The listing builds one solid part. Answer for the finished solid, in the listing's coordinates (mm). A direction names the side the tool comes from. Round coordinates to 2 decimals unless told otherwise and drop trailing zeros. Order: outer loops, then holes, each group sorted by start corner. A loop starts at its lowest first (then second) coordinate and runs counter-clockwise, first axis right, second up. Notation, with made-up numbers: M 53,32.5 L 81,32.5 A18 ccw 81,56.5 Z; hole C 76.25,82.5 d1. An arc over 180 degrees is marked long. Put each result on its own line as item: value. Start each with the question number.
1. The part is cut by section D-D (x = 92). Give the vertices of the cut face in (y, z).
2. The part is cut by section A-A (x = 58.5). Give the vertices of the cut face in (y, z).
3. Consider line 1 (Y direction, x = 32, z = -0.75); line 2 (X direction, y = 49, z = 20.75); line 3 (Z direction, x = 167.5, y = 57). Determine where each line is inside the solid, lowest interval first.
4. Which of the six approach directions +Z, -Z, +X, -X, +Y, -Y give full straight-line access (tool end or side, diameter ignored) to faces 1 (the face through (165.1, 23, 11)), 2 (the face through (-4, 55.88, 21)), 3 (the face through (172.72, 23, 13)), 4 (the face through (-7.62, 23, 13)), 5 (the face through (81, 20, -1.07))?
5. Each of these flat-tipped pins is pushed along its axis until it touches: pin 1 Ø1.2 at (x, z) = (129.5, -0.5) entering from +Y; pin 2 Ø6 at (x, y) = (-13, 12) entering from +Z; pin 3 Ø5 at (x, y) = (115.5, 75.5) entering from -Z; pin 4 Ø1 at (x, y) = (-5, 11) entering from -Z. Where does it stop, or does it pass through?
6. The part is cut by section C-C (y = 34). Give the vertices of the cut face in (x, z), then the cut area to 3 significant figures.
7. The part is cut by section B-B (z = 6.5). Give the vertices of the cut face in (x, y).
from build123d import *

# Parameters (mm, degrees)
SKETCH1_W           = 165.1
SKETCH1_H           = 55.88
BOSS_EXTRUDE1_DEPTH = 2.54
SKETCH1_3_W         = 7.62
SKETCH1_3_H         = 55.88
BOSS_EXTRUDE2_DEPTH = 20
BOSS_EXTRUDE3_DEPTH = 64.2
BOSS_EXTRUDE4_REACH = 127.654
SKETCH3_W           = 2.139816337
SKETCH3_H           = 2.547064604
SKETCH3_H_2         = 2.262901763
SKETCH3_W_2         = 1.069908168
SKETCH3_H_3         = 3.883558818
BOSS_EXTRUDE5_DEPTH = 19.05
BOSS_EXTRUDE6_DEPTH = 2.54
SKETCH6_W           = 26.96027589
SKETCH6_H           = 5.867824753
CUT_EXTRUDE1_DEPTH  = 222.886131721


with BuildPart() as part:
    # Sketch1 → Boss-Extrude1 (new body)
    with BuildSketch(Plane.XY):
        with Locations((82.55, 27.94)):
            Rectangle(SKETCH1_W, SKETCH1_H)
    extrude(amount=BOSS_EXTRUDE1_DEPTH)

    # Sketch1<3> → Boss-Extrude2 (add)
    with BuildSketch(Plane.XY):
        with Locations((-3.81, 27.94)):
            Rectangle(SKETCH1_3_W, SKETCH1_3_H)
        with Locations((168.91, 27.94)):
            Rectangle(SKETCH1_3_W, SKETCH1_3_H)
    extrude(amount=BOSS_EXTRUDE2_DEPTH)

    # Sketch2 → Boss-Extrude3 (add)
    with BuildSketch(Plane(origin=(0, 55.88, 0), x_dir=(1, 0, 0), z_dir=(0, 1, 0))):
        Polygon((165.1, 0), (192.72, 0), (192.72, -2.54), (172.72, -2.54), (172.72, -23), (165.1, -23), align=None)
    boss_extrude3 = extrude(amount=-BOSS_EXTRUDE3_DEPTH)

    # Boss-Extrude4: up to this face of the body (flat: up to its plane)
    boss_extrude4_end = Plane(part.part.faces().sort_by_distance((192.72, 23.78, 1.27))[0])
    # Sketch3 → Boss-Extrude4 (add, up to the picked face)
    with BuildSketch(Plane(origin=(82.55, 0, 0), x_dir=(0, 0, -1), z_dir=(1, 0, 0)), mode=Mode.PRIVATE) as boss_extrude4_sk1:
        with Locations((1.069908169, 54.606467698)):
            Rectangle(SKETCH3_W, SKETCH3_H)
    boss_extrude4_tool1 = split(extrude(boss_extrude4_sk1.sketch, amount=BOSS_EXTRUDE4_REACH, mode=Mode.PRIVATE), bisect_by=boss_extrude4_end, keep=Keep.BOTH, mode=Mode.PRIVATE)
    # Sketch3 → Boss-Extrude4 (add, up to the picked face)
    with BuildSketch(Plane(origin=(82.55, 0, 0), x_dir=(0, 0, -1), z_dir=(1, 0, 0)), mode=Mode.PRIVATE) as boss_extrude4_sk2:
        with Locations((1.069908169, -7.188549119)):
            Rectangle(SKETCH3_W, SKETCH3_H_2)
    boss_extrude4_tool2 = split(extrude(boss_extrude4_sk2.sketch, amount=BOSS_EXTRUDE4_REACH, mode=Mode.PRIVATE), bisect_by=boss_extrude4_end, keep=Keep.BOTH, mode=Mode.PRIVATE)
    # Sketch3 → Boss-Extrude4 (add, up to the picked face)
    with BuildSketch(Plane(origin=(82.55, 0, 0), x_dir=(0, 0, -1), z_dir=(1, 0, 0)), mode=Mode.PRIVATE) as boss_extrude4_sk3:
        with Locations((0.534954084, 20.417406389)):
            Rectangle(SKETCH3_W_2, SKETCH3_H_3)
    boss_extrude4_tool3 = split(extrude(boss_extrude4_sk3.sketch, amount=BOSS_EXTRUDE4_REACH, mode=Mode.PRIVATE), bisect_by=boss_extrude4_end, keep=Keep.BOTH, mode=Mode.PRIVATE)
    boss_extrude4_1 = boss_extrude4_tool1.solids().sort_by(Axis((82.55, 54.606468, -1.069908), (1, 0, 0)))[0]
    add(boss_extrude4_1)
    boss_extrude4_2 = boss_extrude4_tool2.solids().sort_by(Axis((82.55, -7.188549, -1.069908), (1, 0, 0)))[0]
    add(boss_extrude4_2)
    boss_extrude4_3 = boss_extrude4_tool3.solids().sort_by(Axis((82.55, 20.417406, -0.534954), (1, 0, 0)))[0]
    add(boss_extrude4_3)
    boss_extrude4 = boss_extrude4_1 + boss_extrude4_2 + boss_extrude4_3  # Boss-Extrude4 as one shape, for the pattern or mirror that repeats it

    # Mirror1: Boss-Extrude3, Boss-Extrude4 across plane
    add(boss_extrude3.mirror(Plane(origin=(82.55, 0, 0), x_dir=(0, 0, 1), z_dir=(1, 0, 0))))
    add(boss_extrude4.mirror(Plane(origin=(82.55, 0, 0), x_dir=(0, 0, 1), z_dir=(1, 0, 0))))

    # Sketch4 → Boss-Extrude5 (add, symmetric)
    with BuildSketch(Plane(origin=(82.55, 0, 0), x_dir=(0, 0, -1), z_dir=(1, 0, 0))):
        Polygon((-19.210834703, 68.192686786), (-2.54, 55.88), (2.139816337, 55.88), (-16.670834703, 69.773104851), (-16.670834703, 107.873104851), (-19.210834703, 107.873104851), align=None)
    extrude(amount=BOSS_EXTRUDE5_DEPTH, both=True)

    # Sketch5 → Boss-Extrude6 (add)
    with BuildSketch(Plane.XY.offset(19.210834703)):
        Polygon((63.5, 68.192686786), (0, 55.88), (-7.62, 55.88), (63.5, 74.973238457), align=None)
        Polygon((101.6, 74.973238457), (101.6, 68.192686786), (165.1, 55.88), (172.72, 55.88), align=None)
    extrude(amount=-BOSS_EXTRUDE6_DEPTH)

    # Sketch6 → Cut-Extrude1 (cut, through all)
    with BuildSketch(Plane.XY.offset(19.210834703)):
        with Locations((82.391410142, 102.430230737)):
            Rectangle(SKETCH6_W, SKETCH6_H)
    extrude(amount=-CUT_EXTRUDE1_DEPTH, mode=Mode.SUBTRACT)


solid = part.part
Resolved:
1. outline: M -8.32,-2.14 L -6.06,-2.14 L -6.06,0 L -8.32,0 Z; M 0,0 L 18.48,0 L 18.48,-1.07 L 22.36,-1.07 L 22.36,0 L 53.33,0 L 53.33,-2.14 L 55.88,-2.14 L 69.77,16.67 L 99.5,16.67 L 99.5,19.21 L 68.19,19.21 L 55.88,2.54 L 0,2.54 Z; M 105.36,16.67 L 107.87,16.67 L 107.87,19.21 L 105.36,19.21 Z
2. outline: M -8.32,-2.14 L -6.06,-2.14 L -6.06,0 L -8.32,0 Z; M 0,0 L 18.48,0 L 18.48,-1.07 L 22.36,-1.07 L 22.36,0 L 53.33,0 L 53.33,-2.14 L 55.88,-2.14 L 55.88,2.54 L 0,2.54 Z; M 67.22,16.67 L 73.63,16.67 L 73.63,19.21 L 67.22,19.21 Z
3. line 1: -8.32 to -6.06, 18.48 to 22.36, 53.33 to 55.88
3. line 2: -7.62 to 0, 165.1 to 172.72
3. line 3: 16.67 to 19.21
4. face 1: +Z, -Y
4. face 2: +Z, +X, -X, +Y
4. face 3: +Z, +X, +Y, -Y
4. face 4: +Z, -X, +Y, -Y
4. face 5: -Z, +X, -X
5. pin 1: y = 55.88
5. pin 2: z = 2.54
5. pin 3: through
5. pin 4: z = 0
6. outline: M -27.62,0 L 192.72,0 L 192.72,2.54 L 172.72,2.54 L 172.72,23 L 165.1,23 L 165.1,2.54 L 0,2.54 L 0,23 L -7.62,23 L -7.62,2.54 L -27.62,2.54 Z
6. area: 871 mm2
7. outline: M -7.62,-8.32 L 0,-8.32 L 0,55.88 L -7.62,55.88 Z; M 63.5,58.8 L 101.6,58.8 L 101.6,62.26 L 63.5,62.26 Z; M 165.1,-8.32 L 172.72,-8.32 L 172.72,55.88 L 165.1,55.88 Z
